from build123d import *

# Parameters (mm, degrees)
BOSS_EXTRUDE1_DEPTH = 5
SKETCH2_R           = 2.25
CUT_EXTRUDE1_DEPTH  = 6
SKETCH3_W           = 5
SKETCH3_H           = 50
BOSS_EXTRUDE2_DEPTH = 20
SKETCH4_R           = 2.25
CUT_EXTRUDE2_DEPTH  = 36
SKETCH5_W           = 20
SKETCH5_H           = 5
BOSS_EXTRUDE3_DEPTH = 30
CUT_EXTRUDE3_DEPTH  = 38.5
FILLET1_R           = 6
CHAMFER1_SIZE       = 2
FILLET2_R           = 6
FILLET3_R           = 2


with BuildPart() as part:
    # Sketch1 → Boss-Extrude1 (new body)
    with BuildSketch(Plane.XY):
        Polygon((0, 25), (0, 0), (-30, 0), (-30, -12.5), (-55, -12.5), (-55, 37.5), (-30, 37.5), (-30, 25), align=None)
    extrude(amount=BOSS_EXTRUDE1_DEPTH)

    # Sketch2 → Cut-Extrude1 (cut, through all)
    with BuildSketch(Plane.XY.offset(5)):
        with Locations((-45, -2.5)):
            Circle(SKETCH2_R)
        with Locations((-45, 27.5)):
            Circle(SKETCH2_R)
        with BuildLine():
            Line((-10, 10.25), (-20, 10.25))
            ThreePointArc((-20, 10.25), (-22.25, 12.5), (-20, 14.75))
            Line((-20, 14.75), (-10, 14.75))
            ThreePointArc((-10, 14.75), (-7.75, 12.5), (-10, 10.25))
        make_face()
    extrude(amount=-CUT_EXTRUDE1_DEPTH, mode=Mode.SUBTRACT)

    # Sketch3 → Boss-Extrude2 (add)
    with BuildSketch(Plane(origin=(0, 0, 0), x_dir=(-1, 0, 0), z_dir=(0, 0, -1))):
        with Locations((32.5, 12.5)):
            Rectangle(SKETCH3_W, SKETCH3_H)
    extrude(amount=BOSS_EXTRUDE2_DEPTH)

    # Sketch4 → Cut-Extrude2 (cut, through all)
    with BuildSketch(Plane.ZY.offset(35)):
        with Locations((-10, 12.5)):
            Circle(SKETCH4_R)
    extrude(amount=-CUT_EXTRUDE2_DEPTH, mode=Mode.SUBTRACT)

    # Sketch5 → Boss-Extrude3 (add)
    with BuildSketch(Plane(origin=(0, 0, 0), x_dir=(0, 0, -1), z_dir=(1, 0, 0))):
        with Locations((10, 22.5)):
            Rectangle(SKETCH5_W, SKETCH5_H)
        with Locations((10, 2.5)):
            Rectangle(SKETCH5_W, SKETCH5_H)
    extrude(amount=-BOSS_EXTRUDE3_DEPTH)

    # Sketch6 → Cut-Extrude3 (cut, through all)
    with BuildSketch(Plane(origin=(0, 25, 0), x_dir=(1, 0, 0), z_dir=(0, 1, 0))):
        Polygon((-30, 20), (0, 20), (0, 2), (-2.5, 6.5), align=None)
    extrude(amount=-CUT_EXTRUDE3_DEPTH, mode=Mode.SUBTRACT)

    # Fillet1
    fillet1_edges = [part.edges().sort_by_distance(p)[0] for p in [
        (-30, 0, -7.5),
        (-30, 25, -7.5),
    ]]
    fillet(fillet1_edges, radius=FILLET1_R)

    # Chamfer1
    chamfer1_edges = [part.edges().sort_by_distance(p)[0] for p in [
        (-30, 12.5, 0),
        (0, 12.5, 0),
    ]]
    chamfer(chamfer1_edges, length=CHAMFER1_SIZE)

    # Fillet2
    fillet2_edges = [part.edges().sort_by_distance(p)[0] for p in [
        (-55, -12.5, 2.5),
        (-55, 37.5, 2.5),
    ]]
    fillet(fillet2_edges, radius=FILLET2_R)

    # Fillet3
    fillet3_edges = [part.edges().sort_by_distance(p)[0] for p in [
        (0, 25, 1.5),
        (0, 0, 1.5),
        (-30, -12.5, -7.5),
        (-30, 37.5, -7.5),
    ]]
    fillet(fillet3_edges, radius=FILLET3_R)


solid = part.part
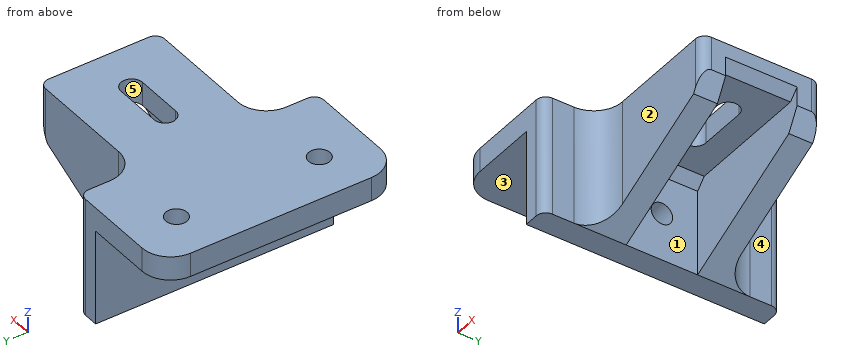
Can you work these out from the model? Positions are in its coordinate system, mm. Face numbers are marked on the shaded views. A direction names the side the tool comes from. Coordinates: 2 decimals unless noted, no trailing zeros. Loops run counter-clockwise (first coordinate to the right, second up) from the corner with the lowest first, then second, coordinate; pieces in that order, holes last. Notation, with made-up numbers: M 46,-6 L 56,-6 A15 cw 56,22 Z; hole C 8.25,83.25 d6. An arc over 180 degrees is marked long. Return JSON: item names as keys, results as strings. Group by question number.
Item 1: Imagine slicing it at D-D (y = 9). Please give me the cut outline in (x, z).
Item 2: I'm going to push flat-ended pins straight in: pin 1 Ø12 at (y, z) = (13, -14) entering from +X; pin 2 Ø3 at (x, z) = (-20, -13.5) entering from -Y; pin 3 Ø1.5 at (y, z) = (4.5, -10.5) entering from -X; pin 4 Ø3.5 at (x, y) = (-45, -2.5) entering from +Z. Where does each tip first touch, or does it pass through?
Item 3: Imagine slicing it at C-C (z = -10.75). Please give me the cut outline in (x, y), and give its area (3 significant figures).
Item 4: Imagine slicing it at A-A (x = -45). Please give me the cut outline in (y, z), and give its area (3 significant figures).
Item 5: Imagine slicing it at B-B (y = -2.5). Please give me the cut outline in (x, z).
Item 6: On a 3-axis mill with a long thin cutter (end or side, diameter ignored), from which of +Z, -Z, +X, -X, +Y, -Y can I reach the whole of each face in a straight line? I mean the marked faces 1, 2, 3, 4 and 5. Say none if no direction works.
Item 7: If I drill on L1, parallel to Y at x = -45, z = 2.1; L2, parallel to Y at x = -23.5, z = -8.5; L3, parallel to Z at x = -37.5, y = 8.5, over which ranges is the centre line in solid material (lowest first)? Write a range as from..to.
Verdict:
{
 "1": {"outline": "M -55,0 L -35,0 L -35,-20 L -30,-20 L -30,-2 L -28,0 L -2,0 L 0,2 L 0,5 L -55,5 Z"},
 "2": {"pin 1": "stops at x = -30", "pin 2": "stops at y = 0", "pin 3": "stops at x = -35", "pin 4": "passes through"},
 "3": {"outline": "M -35,-12.5 L -32,-12.5 A2 ccw -30,-10.5 L -30,-6 A6 cw -24,0 L -11.16,0 L -11.16,5 L -30,5 L -30,10.38 L -35,10.38 Z; M -35,14.62 L -30,14.62 L -30,20 L -11.16,20 L -11.16,25 L -24,25 A6 cw -30,31 L -30,35.5 A2 ccw -32,37.5 L -35,37.5 Z", "area": "431 mm^2"},
 "4": {"outline": "M -12.5,0 L -4.75,0 L -4.75,5 L -12.5,5 Z; M -0.25,0 L 25.25,0 L 25.25,5 L -0.25,5 Z; M 29.75,0 L 37.5,0 L 37.5,5 L 29.75,5 Z", "area": "205 mm^2"},
 "5": {"outline": "M -55,0 L -47.25,0 L -47.25,5 L -55,5 Z; M -42.75,0 L -35,0 L -35,-20 L -30,-20 L -28.87,-19.45 L -28.87,5 L -42.75,5 Z"},
 "6": {"face 1": "-Z, +X", "face 2": "+Z, -Z, +X, -Y", "face 3": "-Z, -X, +Y, -Y", "face 4": "+Z, -Z, +X, +Y", "face 5": "+Z, -Z"},
 "7": {"L1": "y = -12.5..-4.75, -0.25..25.25, 29.75..37.5", "L2": "y = 0..5, 20..25", "L3": "z = 0..5"}
}
